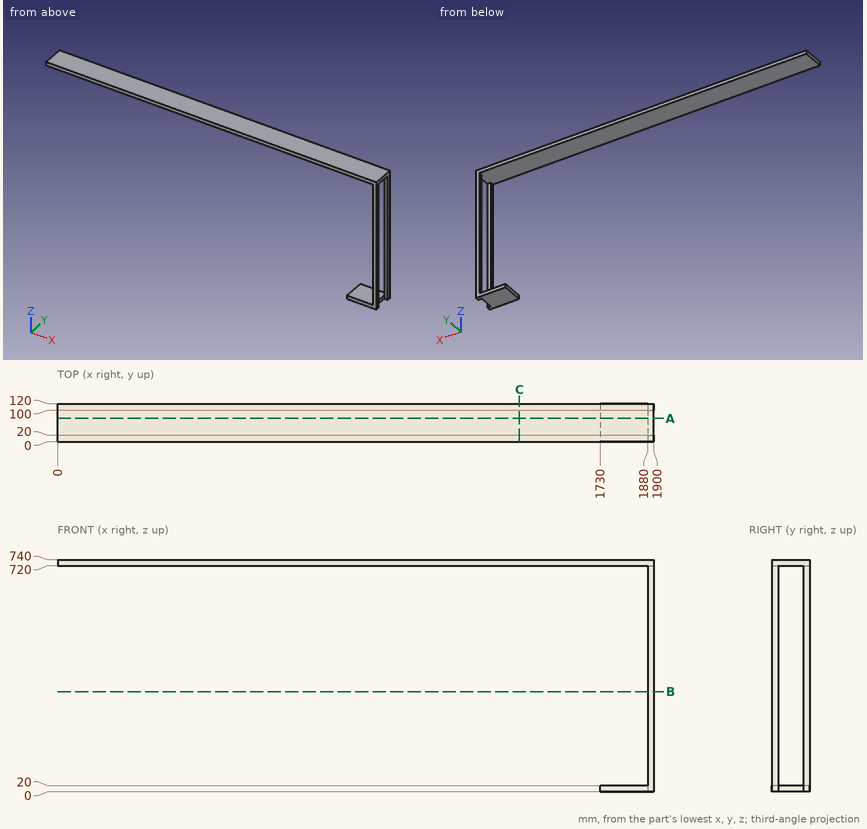
The drawing under review shows one solid part. Ordinate dimensions are in mm from its lowest x, y, z. Give positions to 0.01 mm unless a question says otherwise; leave off trailing zeros. Loops run counter-clockwise (first coordinate to the right, second up) from the corner with the lowest first, then second, coordinate; pieces in that order, holes last. Notation, with made-up numbers: M 73.5,42.25 L 117.5,42.25 A27 ccw 117.5,67.25 Z; hole C -10,29 d9. An arc over 180 degrees is marked long. One line per question, with ' | ' between items. Start each with the question number.
1. Insertion check: P1, Ø16, axis at y = 46.5, z = 13.5, coming from the -X side; P2, Ø10, axis at y = 47.5, z = 6.5, coming from the +X side; P3, Ø1, axis at x = 1317.5, y = 72, coming from the -Z side. Each pin has a flat end and moves straight along its axis. Give the tip position at first contact, or say it passes through.
2. Add section B-B (z = 319.5). Write out the cut boundary in (x, y).
3. To check wall thickness, follow L1, parallel to Z at x = 1769.5, y = 7; L2, parallel to Z at x = 292, y = 89; L3, parallel to X at y = 112.5, z = 265. State the ranges of each line that lie inside material, in increasing order.
4. Add section A-A (y = 74). Write out the cut boundary in (x, z), plus the area to 3 significant figures.
5. Add section C-C (x = 1471.5). Write out the cut boundary in (y, z), plus the area to 3 significant figures.
Worked out:
1) P1: stops at x = 1730 | P2: stops at x = 1880 | P3: stops at z = 720
2) outline: M 1880,0 L 1900,0 L 1900,20 L 1880,20 Z; M 1880,100 L 1900,100 L 1900,120 L 1880,120 Z
3) L1: z = 0 to 20, 720 to 740 | L2: z = 720 to 740 | L3: x = 1880 to 1900
4) outline: M 0,720 L 1900,720 L 1900,740 L 0,740 Z; M 1730,0 L 1880,0 L 1880,20 L 1730,20 Z | area: 41,000 mm²
5) outline: M 0,720 L 120,720 L 120,740 L 0,740 Z | area: 2,400 mm²
